Verification items for the finished model (mm, model axes). Face numbers are marked on the shaded views. A direction names the side the tool comes from. Give positions to 0.01 mm unless a question says otherwise; leave off trailing zeros. Write each loop counter-clockwise with the first axis right and the second up, starting at its lowest first coordinate (ties: lowest second). Pieces come first, ordered by that corner, then holes. Notation, with made-up numbers: M 68.25,7.25 L 105.25,7.25 A21 ccw 105.25,44.25 Z; hole C 25.25,39.5 d11. An arc over 180 degrees is marked long. Write item = value, one per line.
from build123d import *
from build123d import SkipClean  # not in build123d's __all__

# Parameters (mm, degrees)
F0_R       = 25.4
F1_DEPTH   = 6.35
F2_R       = 1.5875
F3_DEPTH   = 3.175
F4_DEPTH   = 1.5875
F5_R       = 1.5875
F3_FACE4_R = 1.5875
F4_FACE_R  = 1.5875
F6_DEPTH   = 1.5875
F7_DEPTH   = 3.175


with BuildPart() as f1:
    # F0 (on Right) → F1 (new body)
    with BuildSketch(Plane.YZ):
        Circle(F0_R)
    extrude(amount=F1_DEPTH)

    # F2 (on face) → F3 (cut)
    with BuildSketch(Plane.YZ.offset(6.35)):
        with BuildLine():
            Line((-3.3675960454, 3.3675960454), (-15.7154482119, 15.7154482119))
            ThreePointArc((-15.7154482119, 15.7154482119), (-20.5332226101, 8.5051392843), (-22.225, 0))
            Line((-22.225, 0), (-4.7625, 0))
            ThreePointArc((-4.7625, 0), (-4.3999762736, 1.8225298466), (-3.3675960454, 3.3675960454))
        make_face()
        with BuildLine():
            ThreePointArc((-15.7154482119, -15.7154482119), (-8.5051392843, -20.5332226101), (0, -22.225))
            Line((0, -22.225), (0, -4.7625))
            ThreePointArc((0, -4.7625), (-1.8225298466, -4.3999762736), (-3.3675960454, -3.3675960454))
            Line((-3.3675960454, -3.3675960454), (-15.7154482119, -15.7154482119))
        make_face()
        with BuildLine():
            ThreePointArc((15.7154482119, -15.7154482119), (20.5332226101, -8.5051392843), (22.225, 0))
            Line((22.225, 0), (4.7625, 0))
            ThreePointArc((4.7625, 0), (4.3999762736, -1.8225298466), (3.3675960454, -3.3675960454))
            Line((3.3675960454, -3.3675960454), (15.7154482119, -15.7154482119))
        make_face()
        with BuildLine():
            Line((3.3675960454, 3.3675960454), (15.7154482119, 15.7154482119))
            ThreePointArc((15.7154482119, 15.7154482119), (8.5051392843, 20.5332226101), (0, 22.225))
            Line((0, 22.225), (0, 4.7625))
            ThreePointArc((0, 4.7625), (1.8225298466, 4.3999762736), (3.3675960454, 3.3675960454))
        make_face()
        Circle(F2_R)
    extrude(amount=-F3_DEPTH, mode=Mode.SUBTRACT)

    # F2 (on face) → F4 (cut)
    with BuildSketch(Plane.YZ.offset(6.35)):
        with BuildLine():
            Line((0, 4.7625), (0, 22.225))
            ThreePointArc((0, 22.225), (-8.5051392843, 20.5332226101), (-15.7154482119, 15.7154482119))
            Line((-15.7154482119, 15.7154482119), (-3.3675960454, 3.3675960454))
            ThreePointArc((-3.3675960454, 3.3675960454), (-1.8225298466, 4.3999762736), (0, 4.7625))
        make_face()
        with BuildLine():
            Line((4.7625, 0), (22.225, 0))
            ThreePointArc((22.225, 0), (20.5332226101, 8.5051392843), (15.7154482119, 15.7154482119))
            Line((15.7154482119, 15.7154482119), (3.3675960454, 3.3675960454))
            ThreePointArc((3.3675960454, 3.3675960454), (4.3999762736, 1.8225298466), (4.7625, 0))
        make_face()
        with BuildLine():
            ThreePointArc((0, -22.225), (8.5051392843, -20.5332226101), (15.7154482119, -15.7154482119))
            Line((15.7154482119, -15.7154482119), (3.3675960454, -3.3675960454))
            ThreePointArc((3.3675960454, -3.3675960454), (1.8225298466, -4.3999762736), (0, -4.7625))
            Line((0, -4.7625), (0, -22.225))
        make_face()
        with BuildLine():
            ThreePointArc((-22.225, 0), (-20.5332226101, -8.5051392843), (-15.7154482119, -15.7154482119))
            Line((-15.7154482119, -15.7154482119), (-3.3675960454, -3.3675960454))
            ThreePointArc((-3.3675960454, -3.3675960454), (-4.3999762736, -1.8225298466), (-4.7625, 0))
            Line((-4.7625, 0), (-22.225, 0))
        make_face()
        with BuildLine():
            ThreePointArc((3.3675960454, -3.3675960454), (4.3999762736, -1.8225298466), (4.7625, 0))
            ThreePointArc((4.7625, 0), (4.3999762736, 1.8225298466), (3.3675960454, 3.3675960454))
            ThreePointArc((3.3675960454, 3.3675960454), (1.8225298466, 4.3999762736), (0, 4.7625))
            ThreePointArc((0, 4.7625), (-1.8225298466, 4.3999762736), (-3.3675960454, 3.3675960454))
            ThreePointArc((-3.3675960454, 3.3675960454), (-4.3999762736, 1.8225298466), (-4.7625, 0))
            ThreePointArc((-4.7625, 0), (-4.3999762736, -1.8225298466), (-3.3675960454, -3.3675960454))
            ThreePointArc((-3.3675960454, -3.3675960454), (-1.8225298466, -4.3999762736), (0, -4.7625))
            ThreePointArc((0, -4.7625), (1.8225298466, -4.3999762736), (3.3675960454, -3.3675960454))
        make_face()
        Circle(F2_R, mode=Mode.SUBTRACT)
    extrude(amount=-F4_DEPTH, mode=Mode.SUBTRACT)

    # F5 (on face) + F3_face (on face) + F3_face1 (on face) + F3_face2 (on face) + F3_face3 (on face) + F3_face4 (on face) + F4_face (on face) → F6 (cut)
    with BuildSketch(Plane(origin=(0, 0, 0), x_dir=(0, -1, 0), z_dir=(-1, 0, 0))):
        with BuildLine():
            Line((3.3675960454, 3.3675960454), (15.7154482119, 15.7154482119))
            ThreePointArc((15.7154482119, 15.7154482119), (8.5051392843, 20.5332226101), (0, 22.225))
            Line((0, 22.225), (0, 4.7625))
            ThreePointArc((0, 4.7625), (1.8225298466, 4.3999762736), (3.3675960454, 3.3675960454))
        make_face()
        with BuildLine():
            ThreePointArc((15.7154482119, -15.7154482119), (20.5332226101, -8.5051392843), (22.225, 0))
            Line((22.225, 0), (4.7625, 0))
            ThreePointArc((4.7625, 0), (4.3999762736, -1.8225298466), (3.3675960454, -3.3675960454))
            Line((3.3675960454, -3.3675960454), (15.7154482119, -15.7154482119))
        make_face()
        with BuildLine():
            ThreePointArc((-15.7154482119, -15.7154482119), (-8.5051392843, -20.5332226101), (0, -22.225))
            Line((0, -22.225), (0, -4.7625))
            ThreePointArc((0, -4.7625), (-1.8225298466, -4.3999762736), (-3.3675960454, -3.3675960454))
            Line((-3.3675960454, -3.3675960454), (-15.7154482119, -15.7154482119))
        make_face()
        with BuildLine():
            Line((-3.3675960454, 3.3675960454), (-15.7154482119, 15.7154482119))
            ThreePointArc((-15.7154482119, 15.7154482119), (-20.5332226101, 8.5051392843), (-22.225, 0))
            Line((-22.225, 0), (-4.7625, 0))
            ThreePointArc((-4.7625, 0), (-4.3999762736, 1.8225298466), (-3.3675960454, 3.3675960454))
        make_face()
        with BuildLine():
            ThreePointArc((3.3675960454, -3.3675960454), (4.3999762736, -1.8225298466), (4.7625, 0))
            ThreePointArc((4.7625, 0), (4.3999762736, 1.8225298466), (3.3675960454, 3.3675960454))
            ThreePointArc((3.3675960454, 3.3675960454), (1.8225298466, 4.3999762736), (0, 4.7625))
            ThreePointArc((0, 4.7625), (-1.8225298466, 4.3999762736), (-3.3675960454, 3.3675960454))
            ThreePointArc((-3.3675960454, 3.3675960454), (-4.3999762736, 1.8225298466), (-4.7625, 0))
            ThreePointArc((-4.7625, 0), (-4.3999762736, -1.8225298466), (-3.3675960454, -3.3675960454))
            ThreePointArc((-3.3675960454, -3.3675960454), (-1.8225298466, -4.3999762736), (0, -4.7625))
            ThreePointArc((0, -4.7625), (1.8225298466, -4.3999762736), (3.3675960454, -3.3675960454))
        make_face()
        Circle(F5_R, mode=Mode.SUBTRACT)
    with BuildSketch(Plane(origin=(3.175, -13.844128687, 5.7344258614), x_dir=(0, 1, 0), z_dir=(1, 0, 0))):
        with BuildLine():
            ThreePointArc((-1.8713195248, 9.9810223505), (-6.689093923, 2.7707134229), (-8.380871313, -5.7344258614))
            Line((-8.380871313, -5.7344258614), (9.081628687, -5.7344258614))
            ThreePointArc((9.081628687, -5.7344258614), (9.4441524134, -3.9118960148), (10.4765326416, -2.366829816))
            Line((10.4765326416, -2.366829816), (-1.8713195248, 9.9810223505))
        make_face()
    with BuildSketch(Plane(origin=(3.175, -5.7344258614, -13.844128687), x_dir=(0, 1, 0), z_dir=(1, 0, 0))):
        with BuildLine():
            ThreePointArc((-9.9810223505, -1.8713195248), (-2.7707134229, -6.689093923), (5.7344258614, -8.380871313))
            Line((5.7344258614, -8.380871313), (5.7344258614, 9.081628687))
            ThreePointArc((5.7344258614, 9.081628687), (3.9118960148, 9.4441524134), (2.366829816, 10.4765326416))
            Line((2.366829816, 10.4765326416), (-9.9810223505, -1.8713195248))
        make_face()
    with BuildSketch(Plane(origin=(3.175, 13.844128687, -5.7344258614), x_dir=(0, 1, 0), z_dir=(1, 0, 0))):
        with BuildLine():
            Line((-10.4765326416, 2.366829816), (1.8713195248, -9.9810223505))
            ThreePointArc((1.8713195248, -9.9810223505), (6.689093923, -2.7707134229), (8.380871313, 5.7344258614))
            Line((8.380871313, 5.7344258614), (-9.081628687, 5.7344258614))
            ThreePointArc((-9.081628687, 5.7344258614), (-9.4441524134, 3.9118960148), (-10.4765326416, 2.366829816))
        make_face()
    with BuildSketch(Plane(origin=(3.175, 5.7344258614, 13.844128687), x_dir=(0, 1, 0), z_dir=(1, 0, 0))):
        with BuildLine():
            ThreePointArc((9.9810223505, 1.8713195248), (2.7707134229, 6.689093923), (-5.7344258614, 8.380871313))
            Line((-5.7344258614, 8.380871313), (-5.7344258614, -9.081628687))
            ThreePointArc((-5.7344258614, -9.081628687), (-3.9118960148, -9.4441524134), (-2.366829816, -10.4765326416))
            Line((-2.366829816, -10.4765326416), (9.9810223505, 1.8713195248))
        make_face()
    with BuildSketch(Plane.YZ.offset(3.175)):
        Circle(F3_FACE4_R)
    with BuildSketch(Plane.YZ.offset(4.7625)):
        with BuildLine():
            Line((-15.7154482119, 15.7154482119), (-3.3675960454, 3.3675960454))
            ThreePointArc((-3.3675960454, 3.3675960454), (-4.3999762736, 1.8225298466), (-4.7625, 0))
            Line((-4.7625, 0), (-22.225, 0))
            ThreePointArc((-22.225, 0), (-20.5332226101, -8.5051392843), (-15.7154482119, -15.7154482119))
            Line((-15.7154482119, -15.7154482119), (-3.3675960454, -3.3675960454))
            ThreePointArc((-3.3675960454, -3.3675960454), (-1.8225298466, -4.3999762736), (0, -4.7625))
            Line((0, -4.7625), (0, -22.225))
            ThreePointArc((0, -22.225), (8.5051392843, -20.5332226101), (15.7154482119, -15.7154482119))
            Line((15.7154482119, -15.7154482119), (3.3675960454, -3.3675960454))
            ThreePointArc((3.3675960454, -3.3675960454), (4.3999762736, -1.8225298466), (4.7625, 0))
            Line((4.7625, 0), (22.225, 0))
            ThreePointArc((22.225, 0), (20.5332226101, 8.5051392843), (15.7154482119, 15.7154482119))
            Line((15.7154482119, 15.7154482119), (3.3675960454, 3.3675960454))
            ThreePointArc((3.3675960454, 3.3675960454), (1.8225298466, 4.3999762736), (0, 4.7625))
            Line((0, 4.7625), (0, 22.225))
            ThreePointArc((0, 22.225), (-8.5051392843, 20.5332226101), (-15.7154482119, 15.7154482119))
        make_face()
        Circle(F4_FACE_R, mode=Mode.SUBTRACT)
    extrude(amount=-F6_DEPTH, dir=(-1, 0, 0), mode=Mode.SUBTRACT)

    # F5 (on face) → F7 (cut)
    with BuildSketch(Plane(origin=(0, 0, 0), x_dir=(0, -1, 0), z_dir=(-1, 0, 0))):
        with BuildLine():
            Line((0, 4.7625), (0, 22.225))
            ThreePointArc((0, 22.225), (-8.5051392843, 20.5332226101), (-15.7154482119, 15.7154482119))
            Line((-15.7154482119, 15.7154482119), (-3.3675960454, 3.3675960454))
            ThreePointArc((-3.3675960454, 3.3675960454), (-1.8225298466, 4.3999762736), (0, 4.7625))
        make_face()
        with BuildLine():
            ThreePointArc((-22.225, 0), (-20.5332226101, -8.5051392843), (-15.7154482119, -15.7154482119))
            Line((-15.7154482119, -15.7154482119), (-3.3675960454, -3.3675960454))
            ThreePointArc((-3.3675960454, -3.3675960454), (-4.3999762736, -1.8225298466), (-4.7625, 0))
            Line((-4.7625, 0), (-22.225, 0))
        make_face()
        with BuildLine():
            ThreePointArc((0, -22.225), (8.5051392843, -20.5332226101), (15.7154482119, -15.7154482119))
            Line((15.7154482119, -15.7154482119), (3.3675960454, -3.3675960454))
            ThreePointArc((3.3675960454, -3.3675960454), (1.8225298466, -4.3999762736), (0, -4.7625))
            Line((0, -4.7625), (0, -22.225))
        make_face()
        with BuildLine():
            Line((4.7625, 0), (22.225, 0))
            ThreePointArc((22.225, 0), (20.5332226101, 8.5051392843), (15.7154482119, 15.7154482119))
            Line((15.7154482119, 15.7154482119), (3.3675960454, 3.3675960454))
            ThreePointArc((3.3675960454, 3.3675960454), (4.3999762736, 1.8225298466), (4.7625, 0))
        make_face()
        Circle(F5_R)
    with SkipClean():  # cleaning this boolean's faces spoils the solid; the shape is the same uncleaned
        extrude(amount=-F7_DEPTH, mode=Mode.SUBTRACT)


solid = f1.part
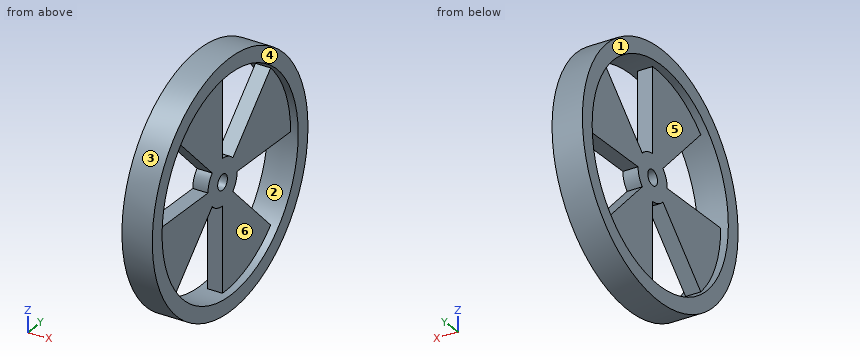
1) Cross-section at C-C on z = 14. Record the boundary of the cut face in (x, y).
From the geometry:
outline = M 0,-21.19 L 6.35,-21.19 L 6.35,-17.26 L 0,-17.26 Z; M 0,17.26 L 1.59,17.26 L 1.59,14 L 4.76,14 L 4.76,17.26 L 6.35,17.26 L 6.35,21.19 L 0,21.19 Z; M 1.59,-14 L 4.76,-14 L 4.76,0 L 1.59,0 Z
2) Material ranges on probe 1 along Z at (x, y) = (4, -8); probe 2 along Y at (x, z) = (4, -6); probe 3 along Y at (x, z) = (4.5, 14), recorded low to high. Write a range as from..to.
From the geometry:
probe_1 = -24.11..-20.74, -8..0, 8..24.11
probe_2 = -24.68..-6, 0..6, 21.4..24.68
probe_3 = -21.19..-17.26, -14..0, 14..21.19
3) Cross-section at D-D on x = 5.5. Record the boundary of the cut face in (y, z) (3 decimals), plus the area to 3 significant figures.
From the geometry:
outline = C 0,0 d50.8; hole C 0,0 d44.45
area = 475 mm^2
4) Depth check by flat-ended pin: P1, Ø3.5, axis at x = 3, y = -14.5, coming from the +Z side; P2, Ø1.6, axis at x = 4, z = 12.5, coming from the +Y side; P3, Ø3.5, axis at x = 2.5, y = 14, coming from the -Z side. Enter the tip coordinate at first touch or a pass-through.
From the geometry:
P1 = 21.97
P2 = 22.54
P3 = -22.25
5) Tool access check on the marked faces 4, 5 and 6. Record the directions out of +Z, -Z, +X, -X, +Y, -Y that give a thin tool (end or side, any length) a straight path to the whole face; none if there is none.
From the geometry:
face_4 = +Z, -Z, +X, +Y, -Y
face_5 = -X
face_6 = +X
6) Draft check along Z on the marked faces 1, 2 and 3. Enter one of: +Z half, -Z half, draft (parallel to the pull), parting line (faces both ways), or undercut.
From the geometry:
face_1 = draft
face_2 = undercut
face_3 = parting line
